```python
from build123d import *

# Parameters (mm, degrees)
SKETCH1_R           = 1.75
BOSS_EXTRUDE1_DEPTH = 4


with BuildPart() as part:
    # Sketch1 → Boss-Extrude1 (new body)
    with BuildSketch(Plane.XY):
        with BuildLine():
            ThreePointArc((13.776114953, 4), (13.893050478, 4.110818553), (14.006628151, 4.225076075))
            ThreePointArc((14.006628151, 4.225076075), (13.913956833, 4.520918628), (13.815037615, 4.814731115))
            ThreePointArc((13.815037615, 4.814731115), (12.481386111, 4.882828881), (11.171803009, 4.621570895))
            ThreePointArc((11.171803009, 4.621570895), (10.939359064, 5.147671635), (10.682156823, 5.662122005))
            ThreePointArc((10.682156823, 5.662122005), (11.718219248, 6.50464102), (12.515850479, 7.575644315))
            ThreePointArc((12.515850479, 7.575644315), (12.35251755, 7.839146011), (12.183637866, 8.099127629))
            ThreePointArc((12.183637866, 8.099127629), (10.874950252, 7.833420336), (9.671482329, 7.254690176))
            ThreePointArc((9.671482329, 7.254690176), (9.315505105, 7.706456036), (8.938444741, 8.140780406))
            ThreePointArc((8.938444741, 8.140780406), (9.7324314, 9.214488384), (10.238655891, 10.450206961))
            ThreePointArc((10.238655891, 10.450206961), (10.01492416, 10.664811019), (9.786695342, 10.874626167))
            ThreePointArc((9.786695342, 10.874626167), (8.585201272, 10.291809183), (7.563466846, 9.431970593))
            ThreePointArc((7.563466846, 9.431970593), (7.1063237, 9.781015462), (6.633097302, 10.107923633))
            ThreePointArc((6.633097302, 10.107923633), (7.135119095, 11.345355554), (7.318128899, 12.668144672))
            ThreePointArc((7.318128899, 12.668144672), (7.048056252, 12.820366729), (6.774818757, 12.966831949))
            ThreePointArc((6.774818757, 12.966831949), (5.756012523, 12.103525808), (4.980210924, 11.016605609))
            ThreePointArc((4.980210924, 11.016605609), (4.450625842, 11.240997714), (3.910967965, 11.439948845))
            ThreePointArc((3.910967965, 11.439948845), (4.089481015, 12.763352309), (3.937776954, 14.090096262))
            ThreePointArc((3.937776954, 14.090096262), (3.638333049, 14.170371647), (3.337255394, 14.244283992))
            ThreePointArc((3.337255394, 14.244283992), (2.565152337, 13.154733392), (2.084030034, 11.909026779))
            ThreePointArc((2.084030034, 11.909026779), (1.515278794, 11.994666739), (0.943098128, 12.053159997))
            ThreePointArc((0.943098128, 12.053159997), (0.786885803, 13.379380698), (0.31, 14.626715284))
            ThreePointArc((0.31, 14.626715284), (0, 14.63), (-0.31, 14.626715284))
            ThreePointArc((-0.31, 14.626715284), (-0.786885803, 13.379380698), (-0.943098128, 12.053159997))
            ThreePointArc((-0.943098128, 12.053159997), (-1.515278794, 11.994666739), (-2.084030034, 11.909026779))
            ThreePointArc((-2.084030034, 11.909026779), (-2.565152337, 13.154733392), (-3.337255394, 14.244283992))
            ThreePointArc((-3.337255394, 14.244283992), (-3.638333049, 14.170371647), (-3.937776954, 14.090096262))
            ThreePointArc((-3.937776954, 14.090096262), (-4.089481015, 12.763352309), (-3.910967965, 11.439948845))
            ThreePointArc((-3.910967965, 11.439948845), (-4.450625842, 11.240997714), (-4.980210924, 11.016605609))
            ThreePointArc((-4.980210924, 11.016605609), (-5.756012523, 12.103525808), (-6.774818757, 12.966831949))
            ThreePointArc((-6.774818757, 12.966831949), (-7.048056252, 12.820366729), (-7.318128899, 12.668144672))
            ThreePointArc((-7.318128899, 12.668144672), (-7.135119095, 11.345355554), (-6.633097302, 10.107923633))
            ThreePointArc((-6.633097302, 10.107923633), (-7.1063237, 9.781015462), (-7.563466846, 9.431970593))
            ThreePointArc((-7.563466846, 9.431970593), (-8.585201272, 10.291809183), (-9.786695342, 10.874626167))
            ThreePointArc((-9.786695342, 10.874626167), (-10.01492416, 10.664811019), (-10.238655891, 10.450206961))
            ThreePointArc((-10.238655891, 10.450206961), (-9.7324314, 9.214488384), (-8.938444741, 8.140780406))
            ThreePointArc((-8.938444741, 8.140780406), (-9.315505105, 7.706456036), (-9.671482329, 7.254690176))
            ThreePointArc((-9.671482329, 7.254690176), (-10.874950252, 7.833420336), (-12.183637866, 8.099127629))
            ThreePointArc((-12.183637866, 8.099127629), (-12.35251755, 7.839146011), (-12.515850479, 7.575644315))
            ThreePointArc((-12.515850479, 7.575644315), (-11.718219248, 6.50464102), (-10.682156823, 5.662122005))
            ThreePointArc((-10.682156823, 5.662122005), (-10.939359064, 5.147671635), (-11.171803009, 4.621570895))
            ThreePointArc((-11.171803009, 4.621570895), (-12.481386111, 4.882828881), (-13.815037615, 4.814731115))
            ThreePointArc((-13.815037615, 4.814731115), (-13.913956833, 4.520918628), (-14.006628151, 4.225076075))
            ThreePointArc((-14.006628151, 4.225076075), (-12.967708283, 3.386083139), (-11.754669706, 2.827691655))
            ThreePointArc((-11.754669706, 2.827691655), (-11.875852861, 2.265440093), (-11.970158218, 1.698061317))
            ThreePointArc((-11.970158218, 1.698061317), (-13.303570578, 1.625431329), (-14.578387742, 1.227807338))
            ThreePointArc((-14.578387742, 1.227807338), (-14.601131037, 0.918625301), (-14.617317864, 0.609030766))
            ThreePointArc((-14.617317864, 0.609030766), (-13.402388515, 0.054765201), (-12.088593461, -0.184412961))
            ThreePointArc((-12.088593461, -0.184412961), (-12.066143147, -0.759137381), (-12.016384363, -1.332143698))
            ThreePointArc((-12.016384363, -1.332143698), (-13.289842779, -1.734098051), (-14.425724151, -2.43626409))
            ThreePointArc((-14.425724151, -2.43626409), (-14.370862478, -2.741388632), (-14.309547736, -3.045282186))
            ThreePointArc((-14.309547736, -3.045282186), (-12.994947386, -3.279993836), (-11.662946429, -3.184930232))
            ThreePointArc((-11.662946429, -3.184930232), (-0.426838607, -12.082462862), (11.409123542, -4))
            Line((11.409123542, -4), (30.75, -4))
            ThreePointArc((30.75, -4), (34.75, 0), (30.75, 4))
            Line((30.75, 4), (13.776114953, 4))
        make_face()
        Circle(SKETCH1_R, mode=Mode.SUBTRACT)
        with Locations((30.75, 0)):
            Circle(SKETCH1_R, mode=Mode.SUBTRACT)
    extrude(amount=BOSS_EXTRUDE1_DEPTH)


solid = part.part
```
CAD build for the part. Positions are in the model's coordinates, mm. A direction names the side the tool comes from. Give positions to 0.01 mm unless a question says otherwise; leave off trailing zeros. Order: outer loops, then holes, each group sorted by start corner. A loop starts at its lowest first (then second) coordinate and runs counter-clockwise, first axis right, second up.
(1) Flat gauge pins, fed straight in: pin 1 (1.5 mm diameter, centred on x = 18, z = 1.5, fed in from -Y); pin 2 (4 mm diameter, centred on x = 21, y = -2, fed in from -Z). Where does each tip first touch, or does it go through?
(2) Saw through at A-A, the plane z = 2.5. State how many separate pieces and enclosed holes the cut face has, then the cut area to 3 significant figures.
(3) Drill centre lines: L1, parallel to Y at x = 0, z = 1.1; L2, parallel to X at y = 0.5, z = 0.6; L3, parallel to Y at x = 30.75, z = 1.5. Where is each one in solid material? Low to high.
(4) Saw through at B-B, the plane x = 23.5. Give the cut face in (y, z).
(5) Mould opens along Y. For faces 1 (the flat face through (21, -4, 2)), 2 (the cylindrical face through (1.523, 11.994, 1.972)), 3 (the cylindrical face through (-7.14, 11.36, 1.97)) say: released by +Y, released by -Y, zero draft, split by the parting line, or undercut.
(6) Tool access for faces 4 (the cylindrical face through (-10.86, 7.83, 1.97)), 5 (the cylindrical face through (-13.42, 0.06, 1.97)), 6 (the flat face through (4, 1, 4)), 7 (the cylindrical face through (5.77, 12.12, 1.97)): list every direction of +Z, -Z, +X, -X, +Y, -Y with a clear straight run to the whole face (end or side of a thin tool).
(7) Saw through at C-C, the plane x = 6. Give the cut face in (y, z).
Results found:
1. pin 1: stops at y = -4
1. pin 2: stops at z = 0
2. separate pieces: 1
2. enclosed holes: 2
2. area: 664 mm2
3. L1: y = -12.09 to -1.75, 1.75 to 14.63
3. L2: x = -14.43 to -1.68, 1.68 to 29.07, 32.43 to 34.72
3. L3: y = -4 to -1.75, 1.75 to 4
4. outline: (-4, 0) - (4, 0) - (4, 4) - (-4, 4) - close
5. face 1: released by -Y
5. face 2: released by +Y
5. face 3: undercut
6. face 4: +Z, -Z
6. face 5: +Z, -Z, -X
6. face 6: +Z, +X, -X, +Y, -Y
6. face 7: +Z, -Z, +Y
7. outline: (-10.5, 0) - (12.35, 0) - (12.35, 4) - (-10.5, 4) - close
